Here's the drawing with two shaded views (mm, measured from the low corner). I have some questions. A direction names the side the tool comes from. Coordinates: 2 decimals unless noted, no trailing zeros. Order: outer loops, then holes, each group sorted by start corner. A loop starts at its lowest first (then second) coordinate and runs counter-clockwise, first axis right, second up. Notation, with made-up numbers: (76, 49) -> (125, 49) arc R21 ccw to (125, 71) -> close; hole circle Ø7 at (-17.75, -22). An arc over 180 degrees is marked (long way). Answer as a JSON object with one key per item and string values. Group by question number.
(1) I need wall thicknesses on line 1 (X direction, y = 28.5, z = 5.5) (3 decimals); line 2 (X direction, y = 28, z = 5). Which ranges of each line are inside material? Lowest first, please.
(2) I want a section at C-C, the plane x = 36.5. List the corners of the cut face in (y, z) for me (3 decimals), plus the area to 3 significant figures.
(3) Which directions (+Z, -Z, +X, -X, +Y, -Y) give clear straight access to the entire face, cutting with the end or side of a thin tool? Please do the marked faces 1 and 2.
(4) I want a section at B-B, the plane y = 50. List the corners of the cut face in (x, z) for me (3 decimals), plus the area to 3 significant figures.
(5) I want a section at D-D, the plane x = 21. List the corners of the cut face in (y, z) for me, plus the area to 3 significant figures.
(6) For pin 1 (1.9 mm diameter, centred on x = 5.5, z = 5.5, fed in from -Y); pin 2 (3 mm diameter, centred on x = 16.5, z = 19, fed in from +Y), each with a flat end and sliding along its axis, tell me the tip position at first contact or that it passes through.
(7) I want a section at A-A, the plane z = 5.5. List the corners of the cut face in (x, y) for me (3 decimals), plus the area to 3 significant figures.
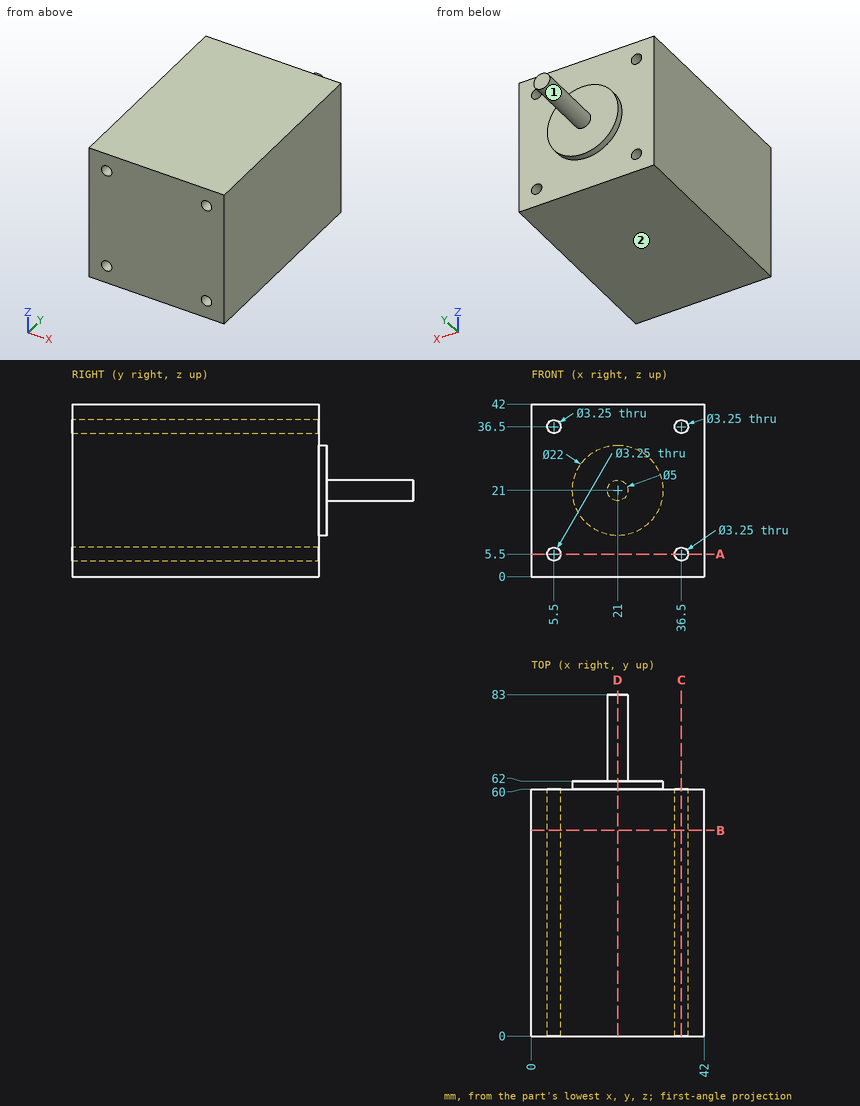
Computed values:
{
 "1": {"line 1": "x = 0 to 3.875, 7.125 to 34.875, 38.125 to 42", "line 2": "x = 0 to 3.95, 7.05 to 34.95, 38.05 to 42"},
 "2": {"outline": "(0, 0) -> (60, 0) -> (60, 3.875) -> (0, 3.875) -> close; (0, 7.125) -> (60, 7.125) -> (60, 34.875) -> (0, 34.875) -> close; (0, 38.125) -> (60, 38.125) -> (60, 42) -> (0, 42) -> close", "area": "2,130 mm2"},
 "3": {"face 1": "+Y", "face 2": "-Z, +X, -X, +Y, -Y"},
 "4": {"outline": "(0, 0) -> (42, 0) -> (42, 42) -> (0, 42) -> close; hole circle Ø3.25 at (5.5, 5.5); hole circle Ø3.25 at (5.5, 36.5); hole circle Ø3.25 at (36.5, 5.5); hole circle Ø3.25 at (36.5, 36.5)", "area": "1,730 mm2"},
 "5": {"outline": "(0, 0) -> (60, 0) -> (60, 10) -> (62, 10) -> (62, 18.5) -> (83, 18.5) -> (83, 23.5) -> (62, 23.5) -> (62, 32) -> (60, 32) -> (60, 42) -> (0, 42) -> close", "area": "2,670 mm2"},
 "6": {"pin 1": "passes through", "pin 2": "stops at y = 62"},
 "7": {"outline": "(0, 0) -> (3.875, 0) -> (3.875, 60) -> (0, 60) -> close; (7.125, 0) -> (34.875, 0) -> (34.875, 60) -> (7.125, 60) -> close; (38.125, 0) -> (42, 0) -> (42, 60) -> (38.125, 60) -> close", "area": "2,130 mm2"}
}
